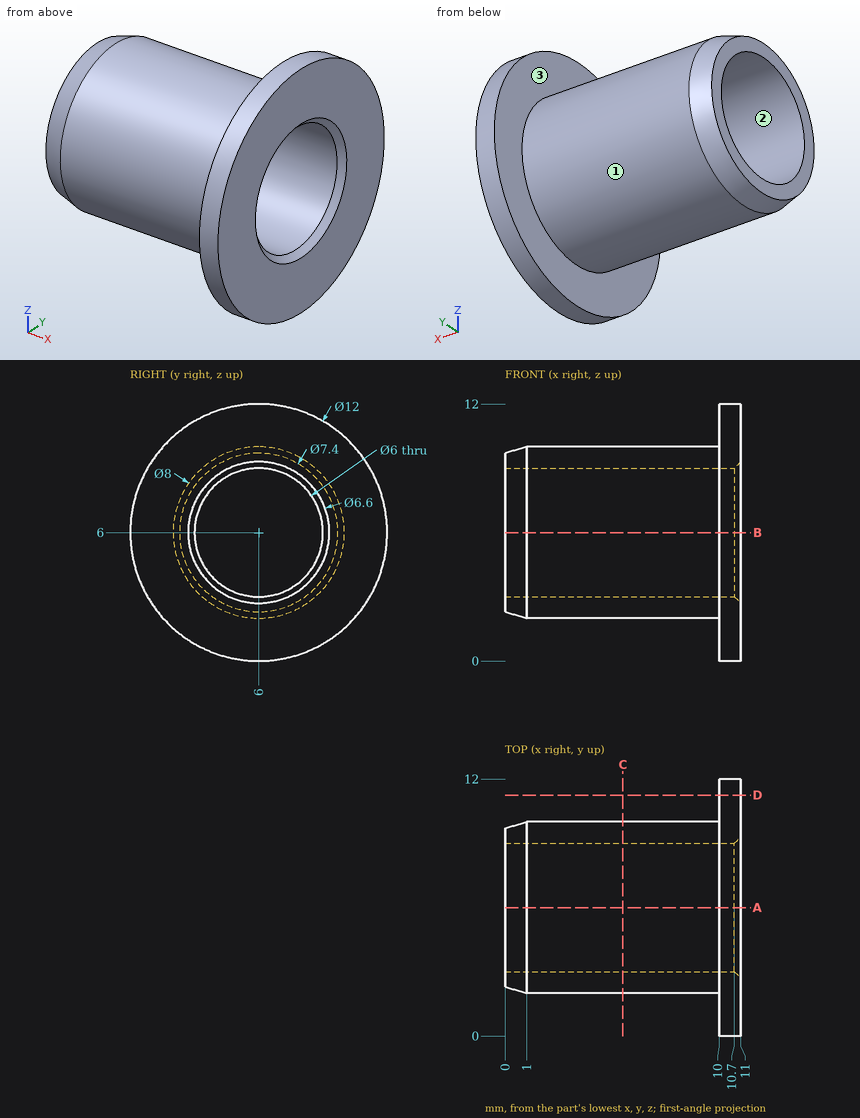
Input: dimensioned drawing with shaded views. Units: mm. Origin: part minimum x, y, z. Coordinates: 2 decimals unless noted, no trailing zeros. Loops run counter-clockwise (first coordinate to the right, second up) from the corner with the lowest first, then second, coordinate; pieces in that order, holes last. Notation, with made-up numbers: (-32, 79) - (25, 79) arc R19 ccw to (25, 90) - close; hole circle Ø5 at (25.5, 53). An arc over 180 degrees is marked (long way). One line per question, with ' | ' between items. Start each with the question number.
(1) Cut plane A-A on y = 6. Output: boundary loops of the cut face in (x, z).
(2) First-contact query: pin 1 (1.5 mm diameter, centred on x = 7.5, z = 2.5, fed in from -Y); pin 2 (6 mm diameter, centred on x = 5.5, z = 9, fed in from +Y); pin 3 (5 mm diameter, centred on x = 6.5, y = 8.5, fed in from +Z); pin 4 (3.5 mm diameter, centred on y = 6, z = 6, fed in from +X). Flat tips, straight axial feed; report the tip coordinate or a pass-through.
(3) Draft query along Z for the marked faces 1, 2 and 3. Return one class per face: +Z half, -Z half, draft (parallel to the pull), parting line (faces both ways), or undercut.
(4) Cut plane C-C on x = 5.5. Output: boundary loops of the cut face in (y, z).
(5) Ray query, L1, parallel to Z at x = 5, y = 6; L2, parallel to Y at x = 6, z = 7.25. Return the intervals inside material, ascending. Write a range as from..to.
(6) Cut plane D-D on y = 11.25. Output: boundary loops of the cut face in (x, z), and give its area (3 significant figures).
Here are the results:
1) outline: (0, 2.3) - (1, 2) - (10, 2) - (10, 0) - (11, 0) - (11, 2.7) - (10.7, 3) - (0, 3) - close; (0, 9) - (10.7, 9) - (11, 9.3) - (11, 12) - (10, 12) - (10, 10) - (1, 10) - (0, 9.7) - close
2) pin 1: y = 3.1 | pin 2: y = 10 | pin 3: z = 10 | pin 4: through
3) face 1: parting line | face 2: undercut | face 3: draft
4) outline: circle Ø8 at (6, 6); hole circle Ø6 at (6, 6)
5) L1: 2..3, 9..10 | L2: 2.2..3.27, 8.73..9.8
6) outline: (10, 3.1) - (11, 3.1) - (11, 8.9) - (10, 8.9) - close | area: 5.81 mm²
